Geometry: final body of the model. Coordinates: model frame, mm. Round coordinates to 2 decimals unless told otherwise and drop trailing zeros. Write each loop counter-clockwise with the first axis right and the second up, starting at its lowest first coordinate (ties: lowest second). Pieces come first, ordered by that corner, then holes. Notation, with made-up numbers: M -6,-20.75 L 10,-20.75 A22 ccw 10,-8.75 Z; hole C 44,23.25 d4. An arc over 180 degrees is marked long. Answer as CSV lines item,"result". Start each with the question number.
Q1. Section query C-C on x = -38. Output: boundary loops of the cut face in (y, z).
Q2. Ray query, probe 1 along Y at (x, z) = (12.7, 2.75); probe 2 along X at (y, z) = (-30.5, 0.75) (3 decimals); probe 3 along X at (y, z) = (-19.25, 2) (3 decimals). Return the intervals inside material, ascending.
Q3. Section query B-B on y = -15.5. Output: boundary loops of the cut face in (x, z).
Q4. Section query A-A on z = 3. Output: boundary loops of the cut face in (x, y) (3 decimals), and give its area (3 significant figures).
Q5. First-contact query: pin 1 (8 mm diameter, centred on x = -45, y = -28, fed in from -Z); pin 2 (1 mm diameter, centred on x = -40, z = 5, fed in from +Y). Flat tips, straight axial feed; report the tip coordinate or a pass-through.
Q6. Section query D-D on y = -36. Output: boundary loops of the cut face in (x, z).
Autodesk Inventor part; units mm, degrees
ref_plane "YZ Plane" through (0, 0, 0) normal (1, 0, 0) x (0, 1, 0)
ref_plane "XZ Plane" through (0, 0, 0) normal (0, 1, 0) x (-1, 0, 0)
ref_plane "XY Plane" through (0, 0, 0) normal (0, 0, 1) x (1, 0, 0)
sketch "Sketch1" plane through (0, 0, 0) normal (0, 0, 1) x (1, 0, 0)
  circle A0 centre (12.7, -31.75) radius 2.1844
  circle A1 centre (-130.175, -31.75) radius 2.1844
  circle A2 centre (-130.175, -19.05) radius 2.1844
  circle A3 centre (12.7, -19.05) radius 2.1844
  line L0 (12.7, -38.1) -> (-130.175, -38.1)
  line L1 (-136.525, -31.75) -> (-136.525, -19.05)
  line L2 (19.05, -19.05) -> (19.05, -31.75)
  arc A4 (-126.1838, -14.1111) -> (-136.525, -19.05) centre (-130.175, -19.05) ccw
  arc A5 (19.05, -19.05) -> (8.7088, -14.1111) centre (12.7, -19.05) ccw
  arc A6 (-23.221, -25.4) -> (8.7088, -14.1111) centre (-23.221, 25.4) ccw
  arc A7 (-126.1838, -14.1111) -> (-94.254, -25.4) centre (-94.254, 25.4) ccw
  arc A8 (12.7, -38.1) -> (19.05, -31.75) centre (12.7, -31.75) ccw
  arc A9 (-136.525, -31.75) -> (-130.175, -38.1) centre (-130.175, -31.75) ccw
  line L3 (-94.254, -25.4) -> (-23.221, -25.4)
  point P0 (0, 0)
  dimension "d0" = 12.7
  dimension "d1" = 6.35
  dimension "d2" = 6.35
  dimension "d3" = 12.7
  dimension "d4" = 50.8
  dimension "d6" = 6.35
extrude "Extrusion1" add sketch "Sketch1" along normal blind 6.35
properties part number "parkbar"
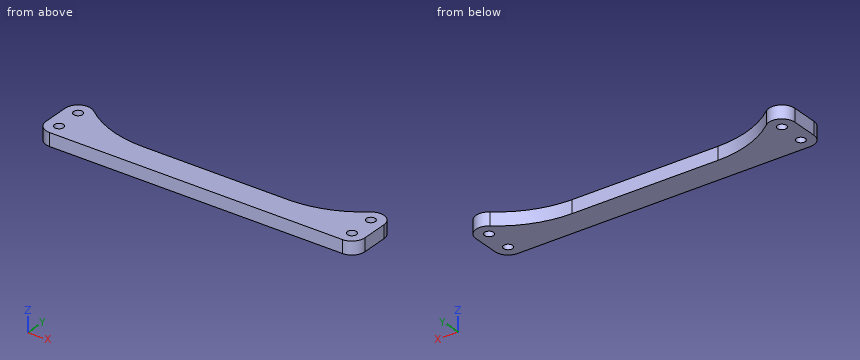
Entries:
1,outline,"M -38.1,0 L -25.4,0 L -25.4,6.35 L -38.1,6.35 Z"
2,probe 1,"y = -38.1 to -33.93, -29.57 to -21.23, -16.87 to -12.7"
2,probe 2,"x = -136.525 to -131.966, -128.384 to 10.909, 14.491 to 19.05"
2,probe 3,"x = -136.525 to -132.35, -128 to -118.482, 1.007 to 10.525, 14.875 to 19.05"
3,outline,"M -135.44,0 L -124.38,0 L -124.38,6.35 L -135.44,6.35 Z; M 6.91,0 L 17.96,0 L 17.96,6.35 L 6.91,6.35 Z"
4,outline,"M -136.525,-31.75 A6.35 ccw -130.175,-38.1 L 12.7,-38.1 A6.35 ccw 19.05,-31.75 L 19.05,-19.05 A6.35 ccw 8.709,-14.111 A50.8 cw -23.221,-25.4 L -94.254,-25.4 A50.8 cw -126.184,-14.111 A6.35 ccw -136.525,-19.05 Z; hole C -130.175,-31.75 d4.369; hole C -130.175,-19.05 d4.369; hole C 12.7,-31.75 d4.369; hole C 12.7,-19.05 d4.369"
4,area,"2,370 mm^2"
5,pin 1,"stops at z = 0"
5,pin 2,"stops at y = -25.4"
6,outline,"M -134.89,0 L 17.42,0 L 17.42,6.35 L -134.89,6.35 Z"
